Can you work these out from the model? Positions are in its coordinate system, mm. Face numbers are marked on the shaded views. A direction names the side the tool comes from. Round coordinates to 2 decimals unless told otherwise and drop trailing zeros. Order: outer loops, then holes, each group sorted by start corner. A loop starts at its lowest first (then second) coordinate and runs counter-clockwise, first axis right, second up. Notation, with made-up numbers: (-12, 65.25) -> (26, 65.25) arc R24 ccw to (26, 100.25) -> close; hole circle Ø5 at (67, -32.5). An arc over 180 degrees is marked (long way). Use a Markdown table: item, result. Add a question column.
Q1. If we section it at D-D on x = -0.25: List the corners of the cut face in (y, z) for me, plus the area to 3 significant figures.
Q2. If we section it at A-A on z = 4.75: List the corners of the cut face in (x, y) for me.
Q3. If we section it at B-B on z = 1.5: List the corners of the cut face in (x, y) for me, plus the area to 3 significant figures.
Q4. For the marked faces 1 and 2, which set-ups out of +Z, -Z, +X, -X, +Y, -Y let a thin tool reach every point of the face, with its end or its side?
Q5. I'm going to push flat-ended pins straight in: pin 1 Ø4 at (x, y) = (2.5, 1) entering from +Z; pin 2 Ø0.6 at (y, z) = (4, -0.5) entering from -X; pin 3 Ø0.5 at (x, y) = (-6.5, 1) entering from -Z. Where does each tip first touch, or does it pass through?
Q6. If we section it at C-C on y = -1: List the corners of the cut face in (x, z) for me, plus the area to 3 significant figures.
Q7. I need wall thicknesses on line 1 along Z through (x, y) = (5, 3); line 2 along X through (y, z) = (4, 4.5); line 3 along X through (y, z) = (2.25, -0.5). Which ranges of each line are inside material? Lowest first, please. Write a range as [from, to].
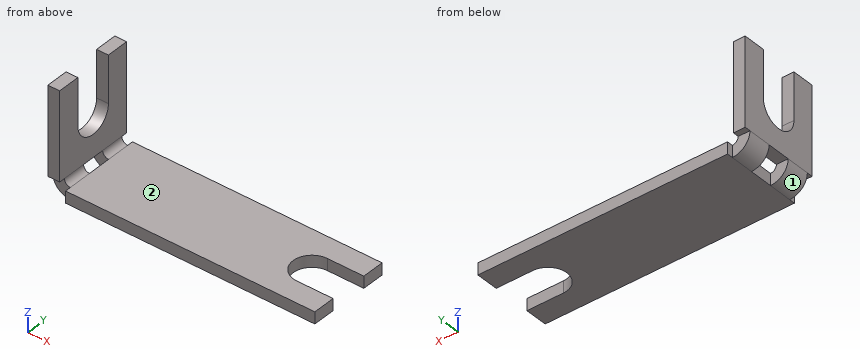
```python
from build123d import *

# Parameters (mm, degrees)
ODGI_CIE_BAZOWE1_DEPTH             = 1
ODGI_CIE_KRAW_DZI1_STRIP_W         = 5
ODGI_CIE_KRAW_DZI1_STRIP_H         = 1
ODGI_CIE_KRAW_DZI1_STRIP_CUT_DEPTH = 7
ODGI_CIE_KRAW_DZI1_DEPTH           = 7
WYTNIJ_WYCI_GNI_CIE1_DEPTH         = 1
WYTNIJ_WYCI_GNI_CIE2_START         = -1.5
SZKIC8_W                           = 4.697403352
SZKIC8_H                           = 2
WYTNIJ_WYCI_GNI_CIE2_DEPTH         = 1.5
WYTNIJ_WYCI_GNI_CIE5_DEPTH         = 0.5
SZKIC7_W                           = 1.5
SZKIC7_H                           = 1.5
WYTNIJ_WYCI_GNI_CIE6_DEPTH         = 0.5


# Sheet-metal steps are written as plain solids
with BuildPart() as part:
    # Szkic1 → Odgięcie bazowe1 (new body)
    with BuildSketch(Plane.XY):
        with BuildLine():
            Line((-5.899587166, 4.522640333), (-5.899587166, -2.477359667))
            Line((-5.899587166, -2.477359667), (15.784981022, -2.477359667))
            Line((15.784981022, -2.477359667), (15.793364792, -0.577359667))
            Line((15.793364792, -0.577359667), (13.620412834, -0.577359667))
            Line((13.620412834, -0.577359667), (12.700412834, -0.577359667))
            ThreePointArc((12.700412834, -0.577359667), (11.100412834, 1.022640333), (12.700412834, 2.622640333))
            Line((12.700412834, 2.622640333), (13.620412834, 2.622640333))
            Line((13.620412834, 2.622640333), (15.807484825, 2.622640333))
            Line((15.807484825, 2.622640333), (15.815868595, 4.522640333))
            Line((15.815868595, 4.522640333), (-5.899587166, 4.522640333))
        make_face()
    extrude(amount=-ODGI_CIE_BAZOWE1_DEPTH)

    # Odgięcie krawędzi1 strip (across the edge) → Odgięcie krawędzi1 strip cut (cut)
    with BuildSketch(Plane(origin=(-5.899587166, 4.522640333, 0), x_dir=(1, 0, 0), z_dir=(0, -1, 0))):
        with Locations((-2, -0.5)):
            Rectangle(ODGI_CIE_KRAW_DZI1_STRIP_W, ODGI_CIE_KRAW_DZI1_STRIP_H)
    extrude(amount=ODGI_CIE_KRAW_DZI1_STRIP_CUT_DEPTH, mode=Mode.SUBTRACT)

    # Odgięcie krawędzi1 section (across the edge) → Odgięcie krawędzi1 (add)
    with BuildSketch(Plane(origin=(-5.899587166, 4.522640333, 0), x_dir=(1, 0, 0), z_dir=(0, -1, 0))):
        with BuildLine():
            Line((-1, 0.5), (-1, 8))
            Line((-1, 8), (0, 8))
            Line((0, 8), (0, 0.5))
            ThreePointArc((0, 0.5), (0.146446609, 0.146446609), (0.5, 0))
            Line((0.5, 0), (0.5, -1))
            ThreePointArc((0.5, -1), (-0.560660172, -0.560660172), (-1, 0.5))
        make_face()
    extrude(amount=ODGI_CIE_KRAW_DZI1_DEPTH)

    # Szkic5 → Wytnij-wyciągnięcie1 (cut)
    with BuildSketch(Plane.ZY.offset(6.899587166)):
        with BuildLine():
            Line((4, -0.577359667), (8, -0.577359667))
            Line((8, -0.577359667), (8, 2.622640333))
            Line((8, 2.622640333), (4, 2.622640333))
            ThreePointArc((4, 2.622640333), (2.4, 1.022640333), (4, -0.577359667))
        make_face()
    extrude(amount=-WYTNIJ_WYCI_GNI_CIE1_DEPTH, mode=Mode.SUBTRACT)

    # Szkic8 → Wytnij-wyciągnięcie2 (cut)
    with BuildSketch(Plane.ZY.offset(6.899587166).offset(WYTNIJ_WYCI_GNI_CIE2_START)):
        with Locations((-1.848701676, 1.022640333)):
            Rectangle(SZKIC8_W, SZKIC8_H)
    extrude(amount=WYTNIJ_WYCI_GNI_CIE2_DEPTH, mode=Mode.SUBTRACT)

    # Szkic6 → Wytnij-wyciągnięcie5 (cut)
    with BuildSketch(Plane.XZ.offset(2.477359667)):
        Polygon((-5.899587166, 0.5), (-5.399587166, 0), (-5.399587166, -1), (-6.899587166, -1), (-6.899587166, 0.5), align=None)
    extrude(amount=-WYTNIJ_WYCI_GNI_CIE5_DEPTH, mode=Mode.SUBTRACT)

    # Szkic7 → Wytnij-wyciągnięcie6 (cut)
    with BuildSketch(Plane(origin=(0, 4.522640333, 0), x_dir=(1, 0, 0), z_dir=(0, 1, 0))):
        with Locations((-6.149587166, 0.25)):
            Rectangle(SZKIC7_W, SZKIC7_H)
    extrude(amount=-WYTNIJ_WYCI_GNI_CIE6_DEPTH, mode=Mode.SUBTRACT)


solid = part.part
```
Answer below:
| question | item | result |
|---|---|---|
| 1 | outline | (-2.48, -1) -> (4.52, -1) -> (4.52, 0) -> (-2.48, 0) -> close |
| 1 | area | 7.00 mm² |
| 2 | outline | (-6.9, -2.48) -> (-5.9, -2.48) -> (-5.9, -0.58) -> (-6.9, -0.58) -> close; (-6.9, 2.62) -> (-5.9, 2.62) -> (-5.9, 4.52) -> (-6.9, 4.52) -> close |
| 3 | outline | (-6.9, -2.48) -> (-5.9, -2.48) -> (-5.9, 4.52) -> (-6.9, 4.52) -> close |
| 3 | area | 7.00 mm² |
| 4 | face 1 | -Z, -X, +Y, -Y |
| 4 | face 2 | +Z, +X, +Y, -Y |
| 5 | pin 1 | z = 0 |
| 5 | pin 2 | x = -6.73 |
| 5 | pin 3 | z = 0.5 |
| 6 | outline | (-6.9, 0.5) arc R1.5 ccw to (-5.4, -1) -> (15.79, -1) -> (15.79, 0) -> (-5.4, 0) arc R0.5 cw to (-5.9, 0.5) -> (-5.9, 8) -> (-6.9, 8) -> close |
| 6 | area | 30.3 mm² |
| 7 | line 1 | [-1, 0] |
| 7 | line 2 | [-6.9, -5.9] |
| 7 | line 3 | [-6.52, 11.67] |
